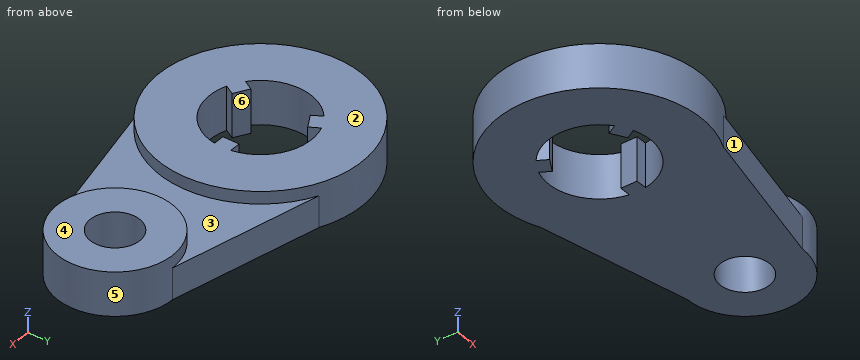
Solid Edge part; units mm, degrees
sketch "Sketch1" plane through (0, 0, 0) normal (0, 0, 1) x (1, 0, 0)
  circle A0 centre (0, 0) radius 41.05
  circle A1 centre (78.21, 0) radius 23.37
  circle A2 centre (0, 0) radius 20.625
  circle A3 centre (78.21, 0) radius 10
extrude "Protrusion1" add sketch "Sketch1" along normal blind 17.73
sketch "Sketch2" plane through (0, 0, 0) normal (0, 0, 1) x (1, 0, 0)
  line L0 (17.5689, 37.1003) -> (30.4967, 0)
  line L1 (30.4967, 0) -> (17.5689, -37.1003)
  line L2 (78.21, -23.37) -> (17.5689, -37.1003)
  line L3 (57, 0) -> (78.21, -23.37)
  line L4 (78.21, 23.37) -> (57, 0)
  line L5 (78.21, 23.37) -> (17.5689, 37.1003)
extrude "ExtrudedProtrusion_3" add sketch "Sketch2" along normal blind 12.71
sketch "Sketch3" plane through (0, 0, 0) normal (0, 0, 1) x (1, 0, 0)
  line L0 (-10.7875, 12.0845) -> (-5.0718, 15.3845)
  line L1 (-7.5718, 19.7147) -> (-5.0718, 15.3845)
  line L2 (-13.2875, 16.4147) -> (-7.5718, 19.7147)
  line L3 (-10.7875, 12.0845) -> (-13.2875, 16.4147)
  line L4 (-5.0718, -15.3845) -> (-10.7875, -12.0845)
  line L5 (-13.2875, -16.4147) -> (-10.7875, -12.0845)
  line L6 (-7.5718, -19.7147) -> (-13.2875, -16.4147)
  line L7 (-5.0718, -15.3845) -> (-7.5718, -19.7147)
  line L8 (20.8593, -3.3) -> (15.8593, -3.3)
  line L9 (15.8593, 3.3) -> (15.8593, -3.3)
  line L10 (15.8593, 3.3) -> (20.8593, 3.3)
  line L11 (20.8593, 3.3) -> (20.8593, -3.3)
extrude "ExtrudedProtrusion_4" add sketch "Sketch3" along normal blind 17.73
Work out the finished part from the listing and answer in its coordinate system (mm). Face numbers are marked on the shaded views. A direction names the side the tool comes from. Give positions to 0.01 mm unless a question says otherwise; leave off trailing zeros. Loops run counter-clockwise (first coordinate to the right, second up) from the corner with the lowest first, then second, coordinate; pieces in that order, holes last. Notation, with made-up numbers: (-24, -20) - (-10, -20) arc R4 ccw to (-10, -16) - close; hole circle Ø7 at (-10.5, -27.5). An arc over 180 degrees is marked (long way). Answer in a Markdown table with one row per item.
(1) Section D-D (x = 22.5) is taken. Give the vertices of the cut face in (y, z).
Results list:
| item | result |
|---|---|
| outline | (-35.98, 0) - (35.98, 0) - (35.98, 12.71) - (34.33, 12.71) - (34.33, 17.73) - (-34.33, 17.73) - (-34.33, 12.71) - (-35.98, 12.71) - close |
(2) Flat-ended cylindrical pins translate along their axes: pin 1 Ø3 at (y, z) = (-8.5, 5.5) entering from -X; pin 2 Ø1 at (x, y) = (20.5, -24) entering from -Z; pin 3 Ø6 at (x, z) = (43, 13.5) entering from -Y; pin 4 Ø4 at (x, z) = (21, 14.5) entering from +Y. Find the tip coordinate at first contact, or state that the pin passes through.
Results list:
| item | result |
|---|---|
| pin 1 | stops at x = -40.45 |
| pin 2 | stops at z = 0 |
| pin 3 | stops at y = -32 |
| pin 4 | stops at y = 36.53 |
(3) Consider L1, parallel to Y at x = 78.21, z = 10.5; L2, parallel to X at y = 15, z = 16; L3, parallel to X at y = -19, z = 13. Determine where each line is inside the solid, lowest interval first. Write a range as [from, to].
Results list:
| item | result |
|---|---|
| L1 | y = [-23.37, -10], [10, 23.37] |
| L2 | x = [-38.21, -14.16], [-12.47, -5.74], [14.16, 38.21], [60.29, 96.13] |
| L3 | x = [-36.39, -7.16], [8.02, 36.39], [64.6, 91.82] |
(4) Section B-B (x = 0) is taken. Give the vertices of the cut face in (y, z) (3 decimals).
Results list:
| item | result |
|---|---|
| outline | (-41.05, 0) - (-20.625, 0) - (-20.625, 17.73) - (-41.05, 17.73) - close; (20.625, 0) - (41.05, 0) - (41.05, 17.73) - (20.625, 17.73) - close |
(5) For a pull along X with two mould halves and no side action, classify the marked faces 1, 2 and 3 as pulls with the +X half, pulls with the -X half, needs draft (parallel to the pull), parting line crosses it, or undercut.
Results list:
| item | result |
|---|---|
| face 1 | pulls with the +X half |
| face 2 | needs draft |
| face 3 | undercut |
(6) Section C-C (y = 0) is taken. Give the vertices of the cut face in (x, z) (3 decimals), and give its area (3 significant figures).
Results list:
| item | result |
|---|---|
| outline | (-41.05, 0) - (-20.625, 0) - (-20.625, 17.73) - (-41.05, 17.73) - close; (15.859, 0) - (68.21, 0) - (68.21, 17.73) - (54.84, 17.73) - (54.84, 12.71) - (41.05, 12.71) - (41.05, 17.73) - (15.859, 17.73) - close; (88.21, 0) - (101.58, 0) - (101.58, 17.73) - (88.21, 17.73) - close |
| area | 1,460 mm² |
(7) A tool of negligible diameter and unlimited length cuts with its end or side. For the marked faces 4, 5 and 6, from which of +Z, -Z, +X, -X, +Y, -Y can it reach the whole face along a straight path? Write none if from no direction.
Results list:
| item | result |
|---|---|
| face 4 | +Z, +X, -X, +Y, -Y |
| face 5 | +Z |
| face 6 | +Z, -Z |
(8) Section A-A (z = 2) is taken. State how many separate pieces and enclosed holes the cut face has, and give its area (3 significant figures).
Results list:
| item | result |
|---|---|
| separate pieces | 1 |
| enclosed holes | 2 |
| area | 7,010 mm² |
